from build123d import *

# Parameters (mm, degrees)
SKETCH_3_W             = 30
SKETCH_3_H             = 1000
EXTRUDE_1_DEPTH        = 100
SKETCH_6_R             = 50
EXTRUDE_2_DEPTH        = 20
PATTERN_LINEAR_1_COUNT = 4
PATTERN_LINEAR_1_PITCH = 250


with BuildPart() as part:
    # 草图3 → 凸台-拉伸1 (new, symmetric)
    with BuildSketch(Plane.XY):
        Rectangle(SKETCH_3_W, SKETCH_3_H)
    extrude(amount=EXTRUDE_1_DEPTH, both=True)

    # 草图6 → 凸台-拉伸2 (add)
    with BuildSketch(Plane.ZY.offset(15)):
        with Locations(Location((0, 375, 0), (0, 0, 90))):
            Circle(SKETCH_6_R)
    extrude_2 = extrude(amount=EXTRUDE_2_DEPTH)

    # 阵列(线性)1: 凸台-拉伸2 ×4
    with Locations(*[(0, -i * PATTERN_LINEAR_1_PITCH, 0) for i in range(1, PATTERN_LINEAR_1_COUNT)]):
        add(extrude_2)


solid = part.part
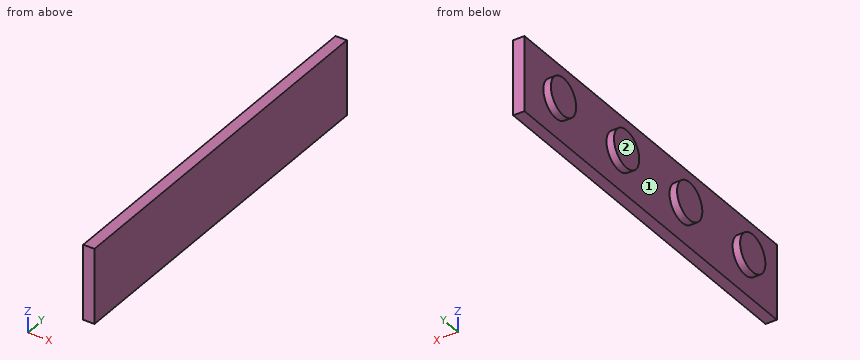
Part model, mm, in its own coordinate system. Face numbers are marked on the shaded views. A direction names the side the tool comes from. Coordinates: 2 decimals unless noted, no trailing zeros. Loops run counter-clockwise (first coordinate to the right, second up) from the corner with the lowest first, then second, coordinate; pieces in that order, holes last. Notation, with made-up numbers: (3.5, 48) - (16.5, 48) arc R18 ccw to (16.5, 57) - close; hole circle Ø10 at (20.25, 68.5). An arc over 180 degrees is marked (long way). Write each question's results on one line, items separated by ' | '. Start each with the question number.
Q1. Slice it at D-D on y = -404.5. Give the cut face in (x, z).
Q2. Drop a flat-ended pin along its axis: pin 1 Ø1 at (x, z) = (-28.5, 0.5) entering from +Y. Give the stop position or say it passes through.
Q3. Slice it at A-A on y = -125. Give the cut face in (x, z).
Q4. Slice it at C-C on z = -41. Give the cut face in (x, y).
Q5. Probe line 1 along Y through (x, z) = (-19.5, -9.5); line 2 along X through (y, z) = (210, -29); line 3 along Z through (x, y) = (-19.5, -413). List the from-to ranges inside material, lowest first.
Q6. Which spindle directions (+Z, -Z, +X, -X, +Y, -Y) get a long thin tool onto all of the face, cutting with end or side? Do the marked faces 1 and 2. Say none if no direction does.
Q7. Slice it at B-B on z = 32. Give the cut face in (x, y), and give its area (3 significant figures).
Answer:
1) outline: (-35, -40.37) - (-15, -40.37) - (-15, -100) - (15, -100) - (15, 100) - (-15, 100) - (-15, 40.37) - (-35, 40.37) - close
2) pin 1: stops at y = 425
3) outline: (-35, -50) - (-15, -50) - (-15, -100) - (15, -100) - (15, 100) - (-15, 100) - (-15, 50) - (-35, 50) - close
4) outline: (-35, -403.62) - (-15, -403.62) - (-15, -500) - (15, -500) - (15, 500) - (-15, 500) - (-15, 403.62) - (-35, 403.62) - (-35, 346.38) - (-15, 346.38) - (-15, 153.62) - (-35, 153.62) - (-35, 96.38) - (-15, 96.38) - (-15, -96.38) - (-35, -96.38) - (-35, -153.62) - (-15, -153.62) - (-15, -346.38) - (-35, -346.38) - close
5) line 1: y = -424.09 to -325.91, -174.09 to -75.91, 75.91 to 174.09, 325.91 to 424.09 | line 2: x = -15 to 15 | line 3: z = -32.5 to 32.5
6) face 1: -X | face 2: +Z, -Z, -X, +Y, -Y
7) outline: (-35, -413.42) - (-15, -413.42) - (-15, -500) - (15, -500) - (15, 500) - (-15, 500) - (-15, 413.42) - (-35, 413.42) - (-35, 336.58) - (-15, 336.58) - (-15, 163.42) - (-35, 163.42) - (-35, 86.58) - (-15, 86.58) - (-15, -86.58) - (-35, -86.58) - (-35, -163.42) - (-15, -163.42) - (-15, -336.58) - (-35, -336.58) - close | area: 36,100 mm2
